from build123d import *

# Parameters (mm, degrees)
EXTRUDE_1_DEPTH     = 450
CUT_EXTRUDE_1_DEPTH = 95
SKETCH_3_R          = 3.5
CUT_EXTRUDE_2_DEPTH = 455.972526643
SKETCH_4_R          = 3.5
CUT_EXTRUDE_3_DEPTH = 455.972526762


with BuildPart() as part:
    # Эскиз1 → Бобышка-Вытянуть1 (new, symmetric)
    with BuildSketch(Plane(origin=(0, 0, 0), x_dir=(0, 1, 0), z_dir=(0, 0, 1))):
        with BuildLine():
            Line((24.75, 30), (-24.75, 30))
            ThreePointArc((-24.75, 30), (-28.462310601, 28.462310601), (-30, 24.75))
            Line((-30, 24.75), (-30, -24.75))
            ThreePointArc((-30, -24.75), (-28.462310601, -28.462310601), (-24.75, -30))
            Line((-24.75, -30), (24.75, -30))
            ThreePointArc((24.75, -30), (28.462310601, -28.462310601), (30, -24.75))
            Line((30, -24.75), (30, 24.75))
            ThreePointArc((30, 24.75), (28.462310601, 28.462310601), (24.75, 30))
        make_face()
        with BuildLine():
            Line((-24.75, -26.5), (24.75, -26.5))
            ThreePointArc((24.75, -26.5), (25.987436867, -25.987436867), (26.5, -24.75))
            Line((26.5, -24.75), (26.5, 24.75))
            ThreePointArc((26.5, 24.75), (25.987436867, 25.987436867), (24.75, 26.5))
            Line((24.75, 26.5), (-24.75, 26.5))
            ThreePointArc((-24.75, 26.5), (-25.987436867, 25.987436867), (-26.5, 24.75))
            Line((-26.5, 24.75), (-26.5, -24.75))
            ThreePointArc((-26.5, -24.75), (-25.987436867, -25.987436867), (-24.75, -26.5))
        make_face(mode=Mode.SUBTRACT)
    extrude(amount=EXTRUDE_1_DEPTH, both=True)

    # Эскиз2 → Вырез-Вытянуть1 (cut)
    with BuildSketch(Plane.XY.offset(450)):
        Polygon((-26.5, 30), (30, 30), (30, -26.5), (-24.75, -26.5), (-26.5, -24.75), align=None)
    extrude(amount=-CUT_EXTRUDE_1_DEPTH, mode=Mode.SUBTRACT)

    # Эскиз3 → Вырез-Вытянуть2 (cut, through all)
    with BuildSketch(Plane.XZ.offset(30)):
        with Locations((0, 400)):
            Circle(SKETCH_3_R)
        with BuildLine():
            Line((23.699747468, 450), (29.699747468, 450))
            Line((29.699747468, 450), (29.699747468, 444))
            ThreePointArc((29.699747468, 444), (27.942388155, 448.242640687), (23.699747468, 450))
        make_face()
    extrude(amount=-CUT_EXTRUDE_2_DEPTH, mode=Mode.SUBTRACT)

    # Эскиз4 → Вырез-Вытянуть3 (cut, through all)
    with BuildSketch(Plane.ZY.offset(30)):
        with Locations(Location((410, 0, 0), (0, 0, 270))):
            Circle(SKETCH_4_R)
        with BuildLine():
            Line((444, 29.699747468), (450, 29.699747468))
            Line((450, 29.699747468), (450, 23.699747468))
            ThreePointArc((450, 23.699747468), (448.242640687, 27.942388155), (444, 29.699747468))
        make_face()
    extrude(amount=-CUT_EXTRUDE_3_DEPTH, mode=Mode.SUBTRACT)


solid = part.part
For this review, take the finished solid that the model builds, in its own axes (mm). A direction names the side the tool comes from. Round coordinates to 2 decimals unless told otherwise and drop trailing zeros. Loops run counter-clockwise (first coordinate to the right, second up) from the corner with the lowest first, then second, coordinate; pieces in that order, holes last. Notation, with made-up numbers: (9, 76) - (58, 76) arc R21 ccw to (58, 97) - close; hole circle Ø9 at (43.25, 2). An arc over 180 degrees is marked (long way). One line per item, written item: value. Start each with the question number.
Item 1: Clearance check with flat-ended pins moving along their axes: pin 1 Ø6.5 at (x, z) = (0, 400) entering from +Y; pin 2 Ø1.5 at (x, z) = (-6, 358) entering from +Y. State where each tip first meets the part, or that it passes through.
Item 2: For L1, parallel to Z at x = 0, y = -27.75; L2, parallel to Y at x = 9.5, z = 211; L3, parallel to Z at x = -28.55, y = 0, list the stretches that pass through material, from the lowest coordinate up.
Item 3: Take a section at A-A (x = -11). Give the boundary of the cut face in (y, z).
Item 4: For faces 1 (the flat face through (27, 14, 355)), 2 (the flat face through (0, 26.5, -42)), 3 (the flat face through (-2, -27, -450)), list the 3-axis set-ups (+Z, -Z, +X, -X, +Y, -Y) from which the entire face can be reached by the end or side of a thin tool; tool diameter is ignored.
Item 5: The part is to be moulded in two halves that separate along Y. For faces 4 (the flat face through (-30, 0, 6)), 5 (the flat face through (0, -30, 6)), 6 (the flat face through (0, 30, -42)), 7 (the flat face through (-26.5, 3, 6)), say which applies: +Y half, -Y half, draft (parallel to the pull), parting line (faces both ways), or undercut.
Item 6: Take a section at B-B (z = 107). Give the boundary of the cut face in (x, y).
Answer below:
1. pin 1: passes through
1. pin 2: stops at y = -26.5
2. L1: z = -450 to 396.5, 403.5 to 450
2. L2: y = -30 to -26.5, 26.5 to 30
2. L3: z = -450 to 406.5, 413.5 to 450
3. outline: (-30, -450) - (-26.5, -450) - (-26.5, 450) - (-30, 450) - close; (26.5, -450) - (30, -450) - (30, 355) - (26.5, 355) - close
4. face 1: +Z, +X, +Y
4. face 2: +Z, -Z
4. face 3: -Z, +X, -X, +Y, -Y
5. face 4: draft
5. face 5: -Y half
5. face 6: +Y half
5. face 7: undercut
6. outline: (-30, -24.75) arc R5.25 ccw to (-24.75, -30) - (24.75, -30) arc R5.25 ccw to (30, -24.75) - (30, 24.75) arc R5.25 ccw to (24.75, 30) - (-24.75, 30) arc R5.25 ccw to (-30, 24.75) - close; hole (-26.5, -24.75) arc R1.75 ccw to (-24.75, -26.5) - (24.75, -26.5) arc R1.75 ccw to (26.5, -24.75) - (26.5, 24.75) arc R1.75 ccw to (24.75, 26.5) - (-24.75, 26.5) arc R1.75 ccw to (-26.5, 24.75) - close
